Here's how the part is built. I have some questions about the finished solid (model axes, mm). Face numbers are marked on the shaded views. A direction names the side the tool comes from. Round coordinates to 2 decimals unless told otherwise and drop trailing zeros. Write each loop counter-clockwise with the first axis right and the second up, starting at its lowest first coordinate (ties: lowest second). Pieces come first, ordered by that corner, then holes. Notation, with made-up numbers: (-17, 3.25) -> (-4, 3.25) arc R11 ccw to (-4, 10.25) -> close; hole circle Ø5 at (51.5, 67). An arc over 180 degrees is marked (long way). Answer as CSV lines item,"result".
Autodesk Inventor part; units mm, degrees
ref_plane "YZ Plane" through (0, 0, 0) normal (1, 0, 0) x (0, 1, 0)
ref_plane "XZ Plane" through (0, 0, 0) normal (0, 1, 0) x (-1, 0, 0)
ref_plane "XY Plane" through (0, 0, 0) normal (0, 0, 1) x (1, 0, 0)
sketch "Sketch1" plane through (0, 0, 0) normal (0, 0, 1) x (1, 0, 0)
  circle A0 centre (0, 0) radius 37.5
  line L0 (0, 0) -> (0, -25)
  circle A1 centre (0, -25) radius 3
  dimension "d0" = 75
  dimension "d1" = 25
  dimension "d2" = 6
extrude "Extrusion1" add sketch "Sketch1" along normal blind 8 contours A0 | A1
sketch "Sketch2" plane through (0, 0, 8) normal (0, 0, 1) x (1, 0, 0)
  line L0 (0, 0) -> (17.6777, 17.6777)
  line L1 (0, 0) -> (25, 0) construction
  circle A0 centre (17.6777, 17.6777) radius 3.15
  circle A1 centre (-17.6777, 17.6777) radius 3.15
  circle A2 centre (-17.6777, -17.6777) radius 3.15
  circle A3 centre (17.6777, -17.6777) radius 3.15
  dimension "d5" = 25
  dimension "d6" = 45
  dimension "d7" = 6.3
  dimension "d10" = 360
extrude "Extrusion2" cut sketch "Sketch2" against normal blind 10
sketch "Sketch3" plane through (0, 0, 8) normal (0, 0, 1) x (1, 0, 0)
  arc A0 (-21.9203, 13.435) -> (-13.435, 21.9203) centre (-17.6777, 17.6777) ccw
  line L0 (-17.6777, 17.6777) -> (-11.6777, 17.6777) construction
  line L1 (-13.435, 21.9203) -> (-19.9189, 28.4042)
  line L2 (-21.9203, 13.435) -> (-28.4042, 19.9189)
  line L3 (-28.4042, 19.9189) -> (-19.9189, 28.4042)
  arc A1 (-13.435, -21.9203) -> (-21.9203, -13.435) centre (-17.6777, -17.6777) ccw
  line L4 (-17.6777, -17.6777) -> (-17.6777, -11.6777) construction
  line L5 (-21.9203, -13.435) -> (-28.4042, -19.9189)
  line L6 (-13.435, -21.9203) -> (-19.9189, -28.4042)
  line L7 (-19.9189, -28.4042) -> (-28.4042, -19.9189)
  arc A2 (21.9203, -13.435) -> (13.435, -21.9203) centre (17.6777, -17.6777) ccw
  line L8 (17.6777, -17.6777) -> (11.6777, -17.6777) construction
  line L9 (13.435, -21.9203) -> (19.9189, -28.4042)
  line L10 (21.9203, -13.435) -> (28.4042, -19.9189)
  line L11 (28.4042, -19.9189) -> (19.9189, -28.4042)
  arc A3 (13.435, 21.9203) -> (21.9203, 13.435) centre (17.6777, 17.6777) ccw
  line L12 (17.6777, 17.6777) -> (17.6777, 11.6777) construction
  line L13 (21.9203, 13.435) -> (28.4042, 19.9189)
  line L14 (13.435, 21.9203) -> (19.9189, 28.4042)
  line L15 (19.9189, 28.4042) -> (28.4042, 19.9189)
  circle A4 centre (0, 0) radius 31.5
  point P0 (-26.1087, 17.6234)
  point P1 (-26.1087, -17.6234)
  point P2 (-17.6234, -26.1087)
  point P3 (17.6234, -26.1087)
  point P4 (26.1087, -17.6234)
  point P5 (26.1087, 17.6234)
  point P6 (17.6234, 26.1087)
  point P7 (-17.6234, 26.1087)
  dimension "d14" = 12
  dimension "d18" = 360
sketch "Sketch4" plane through (0, 0, 0) normal (0, 0, -1) x (-1, 0, 0)
  circle A0 centre (0, 0) radius 42.8826
extrude "Extrusion4" cut sketch "Sketch4" against normal blind 2
sketch "Sketch5" plane through (0, 0, 8) normal (0, 0, 1) x (1, 0, 0)
  line L0 (0, 0) -> (8, 0)
  line L1 (8, 0) -> (8, -40)
  line L2 (8, -40) -> (-8, -40)
  line L3 (-8, -40) -> (-8, 40)
  line L4 (-8, 40) -> (8, 40)
  line L5 (8, 40) -> (8, -40)
  line L6 (0, 0) -> (0, 8)
  line L7 (0, 8) -> (40, 8)
  line L8 (40, 8) -> (40, -8)
  line L9 (40, -8) -> (-40, -8)
  line L10 (-40, -8) -> (-40, 8)
  line L11 (-40, 8) -> (40, 8)
  line L12 (0, 0) -> (0, 40)
  line L13 (0, 40) -> (-5, 40)
  line L14 (-5, 40) -> (5, 40)
  line L15 (5, 40) -> (5, -40)
  line L16 (5, -40) -> (-5, -40)
  line L17 (-5, -40) -> (-5, 40)
  point P0 (8, -8)
  point P1 (8, 8)
  point P2 (-8, 8)
  point P3 (-8, -8)
  dimension "d24" = 8
  dimension "d25" = 40
  dimension "d26" = 16
  dimension "d27" = 80
  dimension "d30" = 90
  dimension "d34" = 5
  dimension "d35" = 10
sketch "Sketch6" plane through (0, 0, 8) normal (0, 0, 1) x (1, 0, 0)
  line L0 (0, 0) -> (0, 40)
  line L1 (0, 40) -> (-5, 40)
  line L2 (-5, 40) -> (5, 40)
  line L3 (5, 40) -> (5, -40)
  line L4 (5, -40) -> (-5, -40)
  line L5 (-5, -40) -> (-5, 40)
  line L6 (0, 0) -> (-40, 0)
  line L7 (-40, 0) -> (-40, -5)
  line L8 (-40, -5) -> (-40, 5)
  line L9 (-40, 5) -> (40, 5)
  line L10 (40, 5) -> (40, -5)
  line L11 (40, -5) -> (-40, -5)
  circle A0 centre (0, 0) radius 37.5
  point P0 (5, -5)
  point P1 (5, 5)
  point P2 (-5, 5)
  point P3 (-5, -5)
  point P4 (37.1652, 5)
  point P5 (5, 37.1652)
  point P6 (-5, 37.1652)
  point P7 (-37.1652, 5)
  point P8 (-37.1652, -5)
  point P9 (-5, -37.1652)
  point P10 (5, -37.1652)
  point P11 (37.1652, -5)
  dimension "d36" = 40
  dimension "d37" = 5
  dimension "d38" = 10
  dimension "d39" = 80
  dimension "d42" = 90
  dimension "d46" = 75
extrude "Extrusion7" add sketch "Sketch6" along normal blind 30 contours L6 L5 L9 L0 | L0 L9 L3 L11 L5 L6 | L9 L5 A0 L0 | L0 A0 L3 L9 | L6 A0 L9 L5 | L5 L11 A0 L6 | L9 A0 L11 L3 | L11 L3 A0 L5
sketch "Sketch7" plane through (5, 5, 8) normal (0, 1, 0) x (1, 0, 0)
  line L0 (0, 0) -> (0, -30)
  line L1 (0, 0) -> (-5, 0)
  line L2 (-5, 0) -> (25, 0)
  line L3 (0, 0) -> (32.1652, 0)
  line L4 (25, 0) -> (25, -14)
  circle A0 centre (25, -14) radius 1.65
  point P0 (-5, 8)
  dimension "d49" = 5
  dimension "d50" = 30
  dimension "d51" = 14
  dimension "d52" = 3.3
extrude "Extrusion8" cut sketch "Sketch7" against normal blind 20
ref_plane "Work Plane1" through (5, 0, 8) normal (0, 1, 0) x (1, 0, 0)
ref_plane "Work Plane2" through (0, 5, 8) normal (1, 0, 0) x (0, 0, -1)
pattern_circular "Circular Pattern2" count 2 over 90 about axis through (0, 0, 8) along (0, 0, 1) of "Extrusion8"
sketch "Sketch8" plane through (-37.1652, 5, 8) normal (0, 1, 0) x (1, 0, 0)
  line L0 (32.1652, 0) -> (32.1652, -30)
  line L1 (32.1652, 0) -> (37.1652, 0)
  line L2 (37.1652, 0) -> (5.9902, 0)
  line L3 (22.6375, 0) -> (16.3375, 0)
  line L4 (5.9902, 0) -> (5.9902, -14)
  circle A0 centre (5.9902, -14) radius 2.15
  point P0 (37.1652, 8)
  dimension "d61" = 31.175
  dimension "d62" = 14
  dimension "d63" = 4.3
extrude "Extrusion9" [suppressed]
pattern_circular "Circular Pattern3" count 2 over 360 about axis through (0, 0, 8) along (0, 0, -1) of "Extrusion8"
chamfer "Chamfer1" distance 2 angle 45 1 edges at (-37.5, 0, 2)
sketch "Sketch10" plane through (5, 5, 8) normal (1, 0, 0) x (0, 0, -1)
  line L0 (0, 0) -> (-30, 0)
  line L1 (0, 0) -> (-30, 0)
  line L2 (-30, 0) -> (-30, 35.3175)
  line L3 (-30, 35.3175) -> (0, 35.3175)
  line L4 (0, 35.3175) -> (0, 0)
  line L5 (0, -10) -> (-30, -10)
  line L6 (0, -10) -> (-32.3439, -10)
  line L7 (-32.3439, -10) -> (-32.3439, -45.8466)
  line L8 (-32.3439, -45.8466) -> (0, -45.8466)
  line L9 (0, -45.8466) -> (0, -10)
  point P0 (8, -5)
extrude "Extrusion11" cut sketch "Sketch10" against normal blind 0.12
mirror "Mirror2" about plane through (0, 5, 8) normal (1, 0, 0) of "Extrusion11"
sketch "Sketch11" plane through (37.1652, 5, 38) normal (0, 1, 0) x (1, 0, 0)
  line L0 (-32.2852, 30) -> (-32.2852, 0)
  line L1 (-32.2852, 30) -> (5.1404, 30)
  line L2 (5.1404, 30) -> (5.1404, -1.2125)
  line L3 (5.1404, -1.2125) -> (-32.2852, -1.2125)
  line L4 (-32.2852, -1.2125) -> (-32.2852, 30)
  line L5 (-74.3303, 30) -> (-42.0452, 30)
  line L6 (-42.0452, 30) -> (-76.613, 30)
  line L7 (-76.613, 30) -> (-76.613, -1.2125)
  line L8 (-76.613, -1.2125) -> (-42.0452, -1.2125)
  line L9 (-42.0452, -1.2125) -> (-42.0452, 30)
  point P0 (-37.1652, 38)
extrude "Extrusion12" cut sketch "Sketch11" against normal blind 0.12
mirror "Mirror3" about plane through (5, 0, 8) normal (0, 1, 0) of "Extrusion12"
mirror "Mirror4" about plane through (5, 0, 8) normal (0, 1, 0) of "Extrusion8", "Circular Pattern2"
chamfer "Chamfer4" distance 3 angle 45 8 edges at (21.0306, 4.88, 38) (-21.0306, 4.88, 38) (4.88, -21.0306, 38) (4.88, 21.0306, 38) (-4.88, -21.0306, 38) (-4.88, 21.0306, 38) (21.0306, -4.88, 38) (-21.0306, -4.88, 38)
sketch "Sketch13" plane through (0, 0, 8) normal (0, 0, 1) x (1, 0, 0)
  arc A0 (37.1811, 4.88) -> (4.88, 37.1811) centre (0, 0) ccw
  circle A1 centre (0, 0) radius 37.5
  line L0 (37.1811, 4.88) -> (4.88, 4.88)
  line L1 (4.88, 4.88) -> (4.88, 37.1811)
  line L2 (37.1811, 4.88) -> (4.88, 4.88)
  line L3 (4.88, 4.88) -> (4.88, 37.1811)
  line L4 (4.88, 37.1811) -> (37.1811, 37.1811)
  line L5 (37.1811, 37.1811) -> (37.1811, 4.88)
  circle A2 centre (17.6777, 17.6777) radius 3.15
  circle A3 centre (17.6777, 17.6777) radius 6
  line L6 (0, 0) -> (0, 7.2893)
  line L7 (0, 0) -> (7.7636, 0)
  arc A4 (-4.88, 37.1811) -> (-37.1811, 4.88) centre (0, 0) ccw
  circle A5 centre (0, 0) radius 37.5
  line L8 (-37.1811, 4.88) -> (-4.88, 4.88)
  line L9 (-4.88, 4.88) -> (-4.88, 37.1811)
  line L10 (-37.1811, 4.88) -> (-4.88, 4.88)
  line L11 (-4.88, 4.88) -> (-4.88, 37.1811)
  line L12 (-4.88, 37.1811) -> (-37.1811, 37.1811)
  line L13 (-37.1811, 37.1811) -> (-37.1811, 4.88)
  circle A6 centre (-17.6777, 17.6777) radius 3.15
  circle A7 centre (-17.6777, 17.6777) radius 6
  arc A8 (4.88, -37.1811) -> (37.1811, -4.88) centre (0, 0) ccw
  circle A9 centre (0, 0) radius 37.5
  line L14 (37.1811, -4.88) -> (4.88, -4.88)
  line L15 (4.88, -4.88) -> (4.88, -37.1811)
  line L16 (37.1811, -4.88) -> (4.88, -4.88)
  line L17 (4.88, -4.88) -> (4.88, -37.1811)
  line L18 (4.88, -37.1811) -> (37.1811, -37.1811)
  line L19 (37.1811, -37.1811) -> (37.1811, -4.88)
  circle A10 centre (17.6777, -17.6777) radius 3.15
  circle A11 centre (17.6777, -17.6777) radius 6
  line L20 (0, 0) -> (0, -7.2893)
  arc A12 (-37.1811, -4.88) -> (-4.88, -37.1811) centre (0, 0) ccw
  circle A13 centre (0, 0) radius 37.5
  line L21 (-37.1811, -4.88) -> (-4.88, -4.88)
  line L22 (-4.88, -4.88) -> (-4.88, -37.1811)
  line L23 (-37.1811, -4.88) -> (-4.88, -4.88)
  line L24 (-4.88, -4.88) -> (-4.88, -37.1811)
  line L25 (-4.88, -37.1811) -> (-37.1811, -37.1811)
  line L26 (-37.1811, -37.1811) -> (-37.1811, -4.88)
  circle A14 centre (-17.6777, -17.6777) radius 3.15
  circle A15 centre (-17.6777, -17.6777) radius 6
  arc A16 (1.88, 37.4528) -> (-1.88, 37.4528) centre (0, 0) ccw
  line L27 (1.88, 37.4528) -> (-1.88, 37.4528)
  line L28 (4.88, 37.1811) -> (17.88, 37.1811)
  line L29 (4.88, 37.1811) -> (4.88, 24.0161)
  point P0 (-37.1811, -4.88)
  dimension "d96" = 12
  dimension "d97" = 13
  dimension "d98" = 13.165
extrude "Extrusion14" add sketch "Sketch13" along normal blind 7 contours L0 L1 A0 | A1 L15 L14 | L9 L8 A1 | A1 L21 L22
properties part number "UR5_Mounting_Plate"
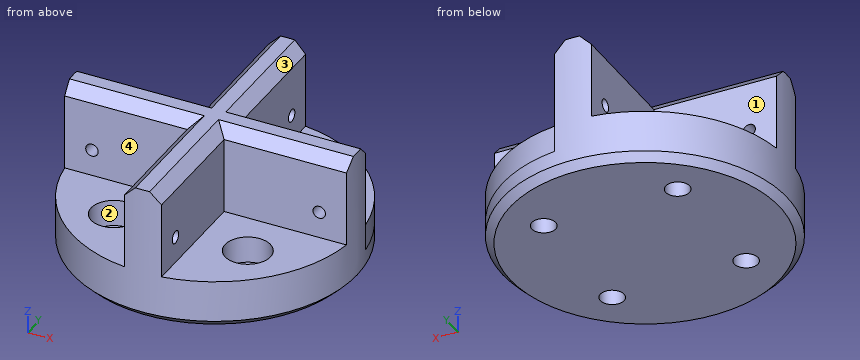
Item 1: Suppose I cut it at C-C, the plane z = 9.5. List the corners of the cut face in (x, y) for me, then the cut area to 3 significant figures.
Results found:
outline,"circle Ø75 at (0, 0); hole circle Ø12 at (-17.68, -17.68); hole circle Ø12 at (-17.68, 17.68); hole circle Ø12 at (17.68, -17.68); hole circle Ø12 at (17.68, 17.68)"
area,"3,970 mm²"
Item 2: For the marked faces 1, 2, 3 and 4, which set-ups out of +Z, -Z, +X, -X, +Y, -Y let a thin tool reach every point of the face, with its end or its side?
Results found:
face 1,"+Z, -X, +Y"
face 2,"+Z"
face 3,"+Z, +X, +Y"
face 4,"+Z, -X, -Y"
Item 3: Will these pins go through, and if not, where does the flat tip stop? pin 1 (7 mm diameter, centred on x = -17.68, y = -17.68, fed in from +Z); pin 2 (6 mm diameter, centred on y = 18, z = 24, fed in from -X); pin 3 (1 mm diameter, centred on x = 3.5, y = 13, fed in from +Z); pin 4 (3 mm diameter, centred on x = 30, z = 22, fed in from -Y).
Results found:
pin 1,"stops at z = 8"
pin 2,"stops at x = -4.88"
pin 3,"stops at z = 36.88"
pin 4,"passes through"
Item 4: Suppose I cut it at B-B, the plane z = 32. List the corners of the cut face in (x, y) for me, then the cut area to 3 significant figures.
Results found:
outline,"(-37.18, -4.88) -> (-4.88, -4.88) -> (-4.88, -37.18) arc R37.5 ccw to (4.88, -37.18) -> (4.88, -4.88) -> (37.18, -4.88) arc R37.5 ccw to (37.18, 4.88) -> (4.88, 4.88) -> (4.88, 37.18) arc R37.5 ccw to (-4.88, 37.18) -> (-4.88, 4.88) -> (-37.18, 4.88) arc R37.5 ccw to start"
area,"1,360 mm²"
Item 5: Suppose I cut it at A-A, the plane z = 22. List the corners of the cut face in (x, y) for me, then the cut area to 3 significant figures.
Results found:
outline,"(-37.18, -4.88) -> (-31.65, -4.88) -> (-31.65, 4.88) -> (-37.18, 4.88) arc R37.5 ccw to start; (-28.35, -4.88) -> (-4.88, -4.88) -> (-4.88, -28.35) -> (4.88, -28.35) -> (4.88, -4.88) -> (28.35, -4.88) -> (28.35, 4.88) -> (4.88, 4.88) -> (4.88, 28.35) -> (-4.88, 28.35) -> (-4.88, 4.88) -> (-28.35, 4.88) -> close; (-4.88, -37.18) arc R37.5 ccw to (4.88, -37.18) -> (4.88, -31.65) -> (-4.88, -31.65) -> close; (-4.88, 31.65) -> (4.88, 31.65) -> (4.88, 37.18) arc R37.5 ccw to (-4.88, 37.18) -> close; (31.65, -4.88) -> (37.18, -4.88) arc R37.5 ccw to (37.18, 4.88) -> (31.65, 4.88) -> close"
area,"1,240 mm²"
Item 6: Suppose I cut it at D-D, the plane z = 36.5. List the corners of the cut face in (x, y) for me.
Results found:
outline,"(-37.35, -3.38) -> (-3.38, -3.38) -> (-3.38, -37.35) arc R37.5 ccw to (3.38, -37.35) -> (3.38, -3.38) -> (37.35, -3.38) arc R37.5 ccw to (37.35, 3.38) -> (3.38, 3.38) -> (3.38, 37.35) arc R37.5 ccw to (-3.38, 37.35) -> (-3.38, 3.38) -> (-37.35, 3.38) arc R37.5 ccw to start"
Item 7: I need wall thicknesses on L1, parallel to Z at x = -30, y = 0.5; L2, parallel to Y at x = 6.5, z = 19.5. Which ranges of each line are inside material? Lowest first, please.
Results found:
L1,"z = 2 to 20.35, 23.65 to 38"
L2,"y = -4.88 to 4.88"
